Verification items for this drawing (mm, ordinates from the low corner). A direction names the side the tool comes from. Give positions to 0.01 mm unless a question says otherwise; leave off trailing zeros. Loops run counter-clockwise (first coordinate to the right, second up) from the corner with the lowest first, then second, coordinate; pieces in that order, holes last. Notation, with made-up numbers: (32.5, 82.5) -> (60.5, 82.5) arc R24 ccw to (60.5, 104.5) -> close; hole circle Ø3 at (-40, 65). An arc over 180 degrees is marked (long way). Write each question's results on one line, items separated by ' | '. Start each with the question number.
Item 1: Cross-section at C-C on x = 10. State how many separate pieces and enclosed holes the cut face has, then the cut area to 3 significant figures.
Item 2: Scan lines: line 1 along X through (y, z) = (8.75, 18); line 2 along Z through (x, y) = (11.5, 3); line 3 along Z through (x, y) = (7.75, 28). Record each from-to range of solid material in increasing order.
Item 3: Cross-section at D-D on z = 18. Enter the section's corners in (x, y).
Item 4: Mould release check, pull along X, two halves, no side actions. Record for the marked faces 1, 2, 3 and 4: pulls with the +X half, pulls with the -X half, needs draft (parallel to the pull), parting line crosses it, or undercut.
Item 5: Access from +Z, -Z, +X, -X, +Y, -Y to the whole of each face (thin tool, end or side, straight path). Record for the marked faces 5, 6 and 7.
Item 6: Gauge pin test, flat ends, axial feed: pin 1 Ø3.5 at (x, z) = (10, 18) entering from -Y; pin 2 Ø4 at (x, y) = (7, 14) entering from -Z; pin 3 Ø12 at (x, y) = (16, 25) entering from +Z. Record the tip position at first contact, or that the pin passes through.
Item 7: Cross-section at A-A on z = 5. Enter the section's corners in (x, y), then the cut area to 3 significant figures.
Item 8: Cross-section at B-B on y = 25. Enter the section's corners in (x, z).
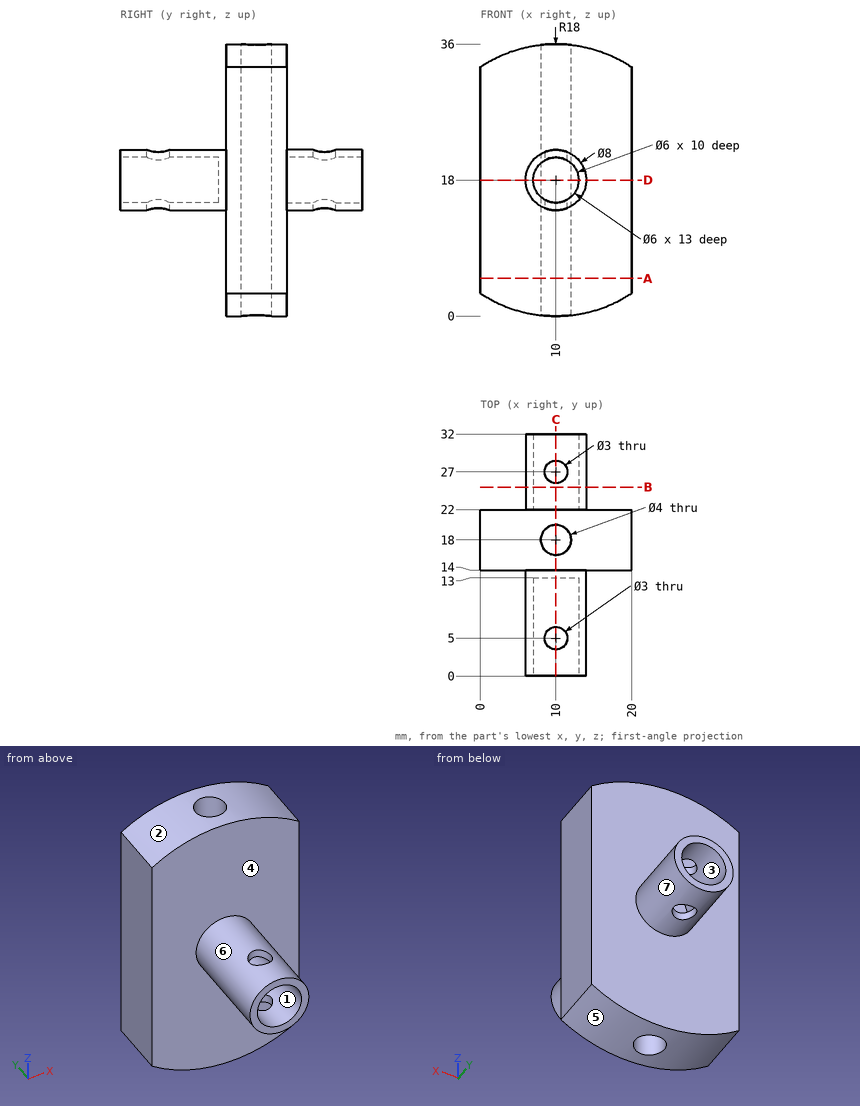
Answer sheet:
1) separate pieces: 6 | enclosed holes: 0 | area: 186 mm²
2) line 1: x = 6 to 7, 13 to 14 | line 2: z = 14.29 to 15.4, 20.6 to 21.71 | line 3: z = 14.69 to 16.02, 19.98 to 21.31
3) outline: (0, 14) -> (6, 14) -> (6, 0) -> (7, 0) -> (7, 13) -> (13, 13) -> (13, 0) -> (14, 0) -> (14, 14) -> (20, 14) -> (20, 22) -> (14, 22) -> (14, 32) -> (13, 32) -> (13, 22) -> (7, 22) -> (7, 32) -> (6, 32) -> (6, 22) -> (0, 22) -> close; hole circle Ø4 at (10, 18)
4) face 1: undercut | face 2: parting line crosses it | face 3: undercut | face 4: needs draft
5) face 5: -Z, +Y, -Y | face 6: -Y | face 7: +Y
6) pin 1: stops at y = 13 | pin 2: stops at z = 0.03 | pin 3: stops at z = 35.98
7) outline: (0, 14) -> (20, 14) -> (20, 22) -> (0, 22) -> close; hole circle Ø4 at (10, 18) | area: 147 mm²
8) outline: circle Ø8 at (10, 18); hole circle Ø6 at (10, 18)
